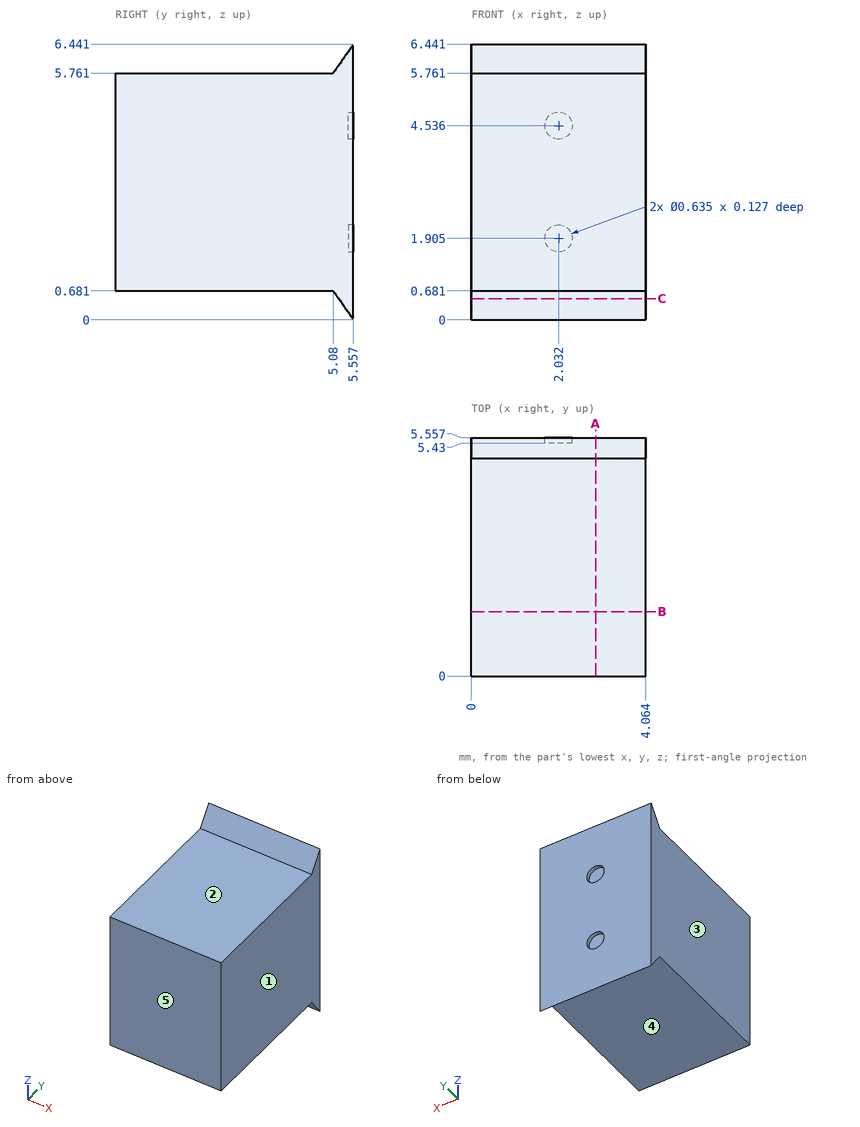
Can you work these out from the drawing? Everything is in mm from the part's minimum corner. A direction names the side the tool comes from. Coordinates: 2 decimals unless noted, no trailing zeros. Write each loop counter-clockwise with the first axis right and the second up, starting at its lowest first coordinate (ties: lowest second). Pieces come first, ordered by that corner, then holes. Notation, with made-up numbers: (-18, -14) -> (11, -14) arc R8 ccw to (11, -1) -> close; hole circle Ø5 at (62.5, 64). An arc over 180 degrees is marked (long way). Write each question's results on one line, items separated by ' | '. Start each with the question number.
Item 1: Please list where these lines run through material, in increasing order: probe 1 along Z at (x, y) = (1.8, 2.5); probe 2 along Y at (x, z) = (2.3, 2); probe 3 along Y at (x, z) = (2.3, 0.5) (1 decimal).
Item 2: If we section it at C-C, the plane z = 0.5: Write out the boundary of the cut face in (x, y).
Item 3: On a 3-axis mill with a long thin cutter (end or side, diameter ignored), from which of +Z, -Z, +X, -X, +Y, -Y can I reach the whole of each face in a straight line? I mean the marked faces 4 and 5. Say none if no direction works.
Item 4: I'm going to push flat-ended pins straight in: P1, Ø1.5, axis at x = 3.5, z = 3, coming from the -Y side; P2, Ø1.5, axis at x = 3, y = 2.5, coming from the -Z side. Where does each tip first touch, or does it pass through?
Item 5: If we section it at B-B, the plane y = 1.5: Write out the boundary of the cut face in (x, z).
Item 6: If we section it at A-A, the plane x = 2.9: Write out the boundary of the cut face in (y, z).
Item 7: Thinking about a two-plate mould opening in X: for the marked faces 1, 2 and 3, which applies, released by +X, released by -X, zero draft, split by the parting line, or undercut?
Answer block:
1) probe 1: 0.68 to 5.76 | probe 2: 0 to 5.43 | probe 3: 5.2 to 5.6
2) outline: (0, 5.21) -> (4.06, 5.21) -> (4.06, 5.56) -> (0, 5.56) -> close
3) face 4: -Z, +X, -X, -Y | face 5: +Z, -Z, +X, -X, -Y
4) P1: y = 0 | P2: z = 0.68
5) outline: (0, 0.68) -> (4.06, 0.68) -> (4.06, 5.76) -> (0, 5.76) -> close
6) outline: (0, 0.68) -> (5.08, 0.68) -> (5.56, 0) -> (5.56, 6.44) -> (5.08, 5.76) -> (0, 5.76) -> close
7) face 1: released by +X | face 2: zero draft | face 3: released by -X
